from build123d import *

# Parameters (mm, degrees)
F0_W     = 1.1863263941
F0_H     = 11.1158097386
F0_R     = 4
F1_DEPTH = 3


with BuildPart() as f1:
    # F0 (on Top) → F1 (new body)
    with BuildSketch(Plane.XY):
        with BuildLine():
            ThreePointArc((26.4942798836, 5.2664663043), (23.5653476954, 12.3375341161), (16.4942798836, 15.2664663043))
            Line((16.4942798836, 15.2664663043), (-16.4942798836, 15.2664663043))
            ThreePointArc((-16.4942798836, 15.2664663043), (-23.5653476954, 12.3375341161), (-26.4942798836, 5.2664663043))
            Line((-26.4942798836, 5.2664663043), (-26.4942798836, -5.2664663043))
            ThreePointArc((-26.4942798836, -5.2664663043), (-23.5653476954, -12.3375341161), (-16.4942798836, -15.2664663043))
            Line((-16.4942798836, -15.2664663043), (16.4942798836, -15.2664663043))
            ThreePointArc((16.4942798836, -15.2664663043), (23.5653476954, -12.3375341161), (26.4942798836, -5.2664663043))
            Line((26.4942798836, -5.2664663043), (26.4942798836, 5.2664663043))
        make_face()
        with BuildLine():
            Line((-15.0588020888, -5.2664663043), (-15.0588020888, 5.1773203903))
            Line((-15.0588020888, 5.1773203903), (-12.107843756, 5.1773203903))
            add(Edge.make_bspline(
                [(-12.107843756, 5.1773203903), (-10.0300582219, 5.1773203903), (-9.1008835028, 4.5555847849)],
                knots=[0, 0, 0, 1, 1, 1], degree=2))
            add(Edge.make_bspline(
                [(-9.1008835028, 4.5555847849), (-8.1717087838, 3.9338491795), (-8.1717087838, 2.5920888841)],
                knots=[0, 0, 0, 1, 1, 1], degree=2))
            add(Edge.make_bspline(
                [(-8.1717087838, 2.5920888841), (-8.1717087838, 1.6617712688), (-8.6894408228, 1.0583220047)],
                knots=[0, 0, 0, 1, 1, 1], degree=2))
            add(Edge.make_bspline(
                [(-8.6894408228, 1.0583220047), (-9.2071728618, 0.4548727407), (-10.2014926719, 0.2765809127)],
                knots=[0, 0, 0, 1, 1, 1], degree=2))
            Line((-10.2014926719, 0.2765809127), (-10.2014926719, 0.20572134))
            add(Edge.make_bspline(
                [(-10.2014926719, 0.20572134), (-7.8219825058, -0.2011497547), (-7.8219825058, -2.2949358375)],
                knots=[0, 0, 0, 1, 1, 1], degree=2))
            add(Edge.make_bspline(
                [(-7.8219825058, -2.2949358375), (-7.8219825058, -3.6938409495), (-8.7683006698, -4.4801536269)],
                knots=[0, 0, 0, 1, 1, 1], degree=2))
            add(Edge.make_bspline(
                [(-8.7683006698, -4.4801536269), (-9.7146188339, -5.2664663043), (-11.4152485779, -5.2664663043)],
                knots=[0, 0, 0, 1, 1, 1], degree=2))
            Line((-11.4152485779, -5.2664663043), (-15.0588020888, -5.2664663043))
        make_face(mode=Mode.SUBTRACT)
        with BuildLine():
            add(Edge.make_bspline(
                [(-1.0971804801, -5.2916100236), (-1.6571996834, -5.4104712423), (-2.4503697388, -5.4104712423)],
                knots=[0, 0, 0, 1, 1, 1], degree=2))
            add(Edge.make_bspline(
                [(-2.4503697388, -5.4104712423), (-4.1852863729, -5.4104712423), (-5.1898922499, -4.3521492376)],
                knots=[0, 0, 0, 1, 1, 1], degree=2))
            add(Edge.make_bspline(
                [(-5.1898922499, -4.3521492376), (-6.194498127, -3.2938272328), (-6.194498127, -1.4171914534)],
                knots=[0, 0, 0, 1, 1, 1], degree=2))
            add(Edge.make_bspline(
                [(-6.194498127, -1.4171914534), (-6.194498127, 0.4777306674), (-5.261894719, 1.5920545924)],
                knots=[0, 0, 0, 1, 1, 1], degree=2))
            add(Edge.make_bspline(
                [(-5.261894719, 1.5920545924), (-4.3292913109, 2.7063785175), (-2.7566659561, 2.7063785175)],
                knots=[0, 0, 0, 1, 1, 1], degree=2))
            add(Edge.make_bspline(
                [(-2.7566659561, 2.7063785175), (-1.2869012714, 2.7063785175), (-0.4297290214, 1.7383453231)],
                knots=[0, 0, 0, 1, 1, 1], degree=2))
            add(Edge.make_bspline(
                [(-0.4297290214, 1.7383453231), (0.4274432287, 0.7703121287), (0.4274432287, -0.816027982)],
                knots=[0, 0, 0, 1, 1, 1], degree=2))
            Line((0.4274432287, -0.816027982), (0.4274432287, -1.5657679768))
            Line((0.4274432287, -1.5657679768), (-4.9647416723, -1.5657679768))
            add(Edge.make_bspline(
                [(-4.9647416723, -1.5657679768), (-4.9281689896, -2.9441009548), (-4.2675749089, -3.6584111632)],
                knots=[0, 0, 0, 1, 1, 1], degree=2))
            add(Edge.make_bspline(
                [(-4.2675749089, -3.6584111632), (-3.6069808282, -4.3727213716), (-2.4069396781, -4.3727213716)],
                knots=[0, 0, 0, 1, 1, 1], degree=2))
            add(Edge.make_bspline(
                [(-2.4069396781, -4.3727213716), (-1.1428963334, -4.3727213716), (0.0914317067, -3.8447032655)],
                knots=[0, 0, 0, 1, 1, 1], degree=2))
            Line((0.0914317067, -3.8447032655), (0.0914317067, -4.9030252703))
            add(Edge.make_bspline(
                [(0.0914317067, -4.9030252703), (-0.5371612767, -5.1727488049), (-1.0971804801, -5.2916100236)],
                knots=[0, 0, 0, 1, 1, 1], degree=2))
        make_face(mode=Mode.SUBTRACT)
        with BuildLine():
            Line((15.5456759268, -5.2664663043), (14.6656457501, -5.2664663043))
            Line((14.6656457501, -5.2664663043), (14.4302091054, -4.1509994829))
            Line((14.4302091054, -4.1509994829), (14.3730642888, -4.1509994829))
            add(Edge.make_bspline(
                [(14.3730642888, -4.1509994829), (13.7879013661, -4.8870247216), (13.2061671324, -5.1487479819)],
                knots=[0, 0, 0, 1, 1, 1], degree=2))
            add(Edge.make_bspline(
                [(13.2061671324, -5.1487479819), (12.6244328987, -5.4104712423), (11.7512601, -5.4104712423)],
                knots=[0, 0, 0, 1, 1, 1], degree=2))
            add(Edge.make_bspline(
                [(11.7512601, -5.4104712423), (10.5877916326, -5.4104712423), (9.9271975519, -4.8093077709)],
                knots=[0, 0, 0, 1, 1, 1], degree=2))
            add(Edge.make_bspline(
                [(9.9271975519, -4.8093077709), (9.2666034712, -4.2081442996), (9.2666034712, -3.1018206488)],
                knots=[0, 0, 0, 1, 1, 1], degree=2))
            add(Edge.make_bspline(
                [(9.2666034712, -3.1018206488), (9.2666034712, -0.7314536534), (13.0587335054, -0.61716402)],
                knots=[0, 0, 0, 1, 1, 1], degree=2))
            Line((13.0587335054, -0.61716402), (14.3867790448, -0.5737339594))
            Line((14.3867790448, -0.5737339594), (14.3867790448, -0.0868601213))
            add(Edge.make_bspline(
                [(14.3867790448, -0.0868601213), (14.3867790448, 0.8343143234), (13.9913369134, 1.2731865154)],
                knots=[0, 0, 0, 1, 1, 1], degree=2))
            add(Edge.make_bspline(
                [(13.9913369134, 1.2731865154), (13.5958947821, 1.7120587074), (12.7227219834, 1.7120587074)],
                knots=[0, 0, 0, 1, 1, 1], degree=2))
            add(Edge.make_bspline(
                [(12.7227219834, 1.7120587074), (11.744402722, 1.7120587074), (10.5100746819, 1.1131810287)],
                knots=[0, 0, 0, 1, 1, 1], degree=2))
            Line((10.5100746819, 1.1131810287), (10.1443478552, 2.0206407174))
            add(Edge.make_bspline(
                [(10.1443478552, 2.0206407174), (10.7226533999, 2.3337943128), (11.4118198889, 2.5120861408)],
                knots=[0, 0, 0, 1, 1, 1], degree=2))
            add(Edge.make_bspline(
                [(11.4118198889, 2.5120861408), (12.100986378, 2.6903779688), (12.7958673487, 2.6903779688)],
                knots=[0, 0, 0, 1, 1, 1], degree=2))
            add(Edge.make_bspline(
                [(12.7958673487, 2.6903779688), (14.1947724608, 2.6903779688), (14.8702241938, 2.0697852598)],
                knots=[0, 0, 0, 1, 1, 1], degree=2))
            add(Edge.make_bspline(
                [(14.8702241938, 2.0697852598), (15.5456759268, 1.4491925507), (15.5456759268, 0.0777169507)],
                knots=[0, 0, 0, 1, 1, 1], degree=2))
            Line((15.5456759268, 0.0777169507), (15.5456759268, -5.2664663043))
        make_face(mode=Mode.SUBTRACT)
        with Locations((3.0435329358, 0.291438565)):
            Rectangle(F0_W, F0_H, mode=Mode.SUBTRACT)
        with Locations((6.7442312634, 0.291438565)):
            Rectangle(F0_W, F0_H, mode=Mode.SUBTRACT)
        with Locations((16.4942798836, 8.2664663043)):
            Circle(F0_R, mode=Mode.SUBTRACT)
    extrude(amount=F1_DEPTH)


solid = f1.part
Could you check a few things on this model? Use its own coordinates, in mm. A direction names the side the tool comes from. Give positions to 0.01 mm unless a question says otherwise; leave off trailing zeros. Use CSV: the item, a comma, the result in double quotes. Start each with the question number.
Item 1: I want a section at A-A, the plane x = -4. Give the number of separate pieces and of enclosed holes in the cut face, then the cut area to 3 significant figures.
Item 2: If I drill on line 1 along Y through (x, z) = (-8.5, 2.35); line 2 along Y through (x, z) = (-14.5, 0.2); line 3 along X through (y, z) = (5.5, 0.3), over which ranges is the centre line in solid material (lowest first)?
Item 3: For faces 4 (the face through (0, 15.266, 1)), 5 (the face through (2.45, 0, 1)), which set-ups out of +Z, -Z, +X, -X, +Y, -Y let a thin tool reach every point of the face, with its end or its side?
Item 4: If we mould it in two halves opening along X, with no side actions, what happens to faces 1 (the face through (-23.5, 12.4, 1.5)), 2 (the face through (0, -3, 0)), 3 (the face through (3, 5.849, 1))? For each: pulls with the +X half, pulls with the -X half, needs draft (parallel to the pull), parting line crosses it, or undercut.
Findings:
1,separate pieces,"3"
1,enclosed holes,"0"
1,area,"75.7 mm2"
2,line 1,"y = -15.27 to -4.22, -0.54 to 1.32, 3.93 to 15.27"
2,line 2,"y = -15.27 to -5.27, 5.18 to 15.27"
2,line 3,"x = -26.49 to 2.45, 3.64 to 6.15, 7.34 to 13.61, 19.38 to 26.49"
3,face 4,"+Z, -Z, +X, -X, +Y"
3,face 5,"+Z, -Z"
4,face 1,"pulls with the -X half"
4,face 2,"needs draft"
4,face 3,"undercut"
